Source: CAD feature listing. Evaluate the final solid. Frame: model axes, mm. Give positions to 0.01 mm unless a question says otherwise; leave off trailing zeros. Order: outer loops, then holes, each group sorted by start corner. A loop starts at its lowest first (then second) coordinate and runs counter-clockwise, first axis right, second up. Notation, with made-up numbers: M 89.5,39 L 139.5,39 A17 cw 139.5,61 Z; hole C 6.25,-26.5 d1. An arc over 180 degrees is marked long. Answer in a Markdown table with one row per item. Add a question column.
(1) Section query C-C, the plane x = 6.25. Return loops of the section in (y, z).
(2) Mould query, pull axis X, two halves, no side actions, for faces 1 (the face through (4, 1, 0)), 2 (the face through (4, 2.54, -2)), 3 (the face through (0, 1, -2)). Classes: pulls with the +X half, pulls with the -X half, needs draft (parallel to the pull), parting line crosses it, or undercut.
(3) Section query A-A, the plane y = 4.5. Return loops of the section in (x, z), plus the area to 3 significant figures.
(4) Pin query (flat end, axial travel): P1, Ø0.7, axis at y = 4, z = -1, coming from the -X side; P2, Ø0.7, axis at y = 6.5, z = -3.5, coming from the +X side; P3, Ø1.5, axis at x = 6, y = 3, coming from the +Z side; P4, Ø3, axis at x = 3, y = 6.5, coming from the +Z side. Return the tip coordinate at first contact, or that it passes through.
(5) Material intervals for line 1 along X through (y, z) = (6.5, -3.4); line 2 along Y through (x, z) = (6.75, -3.1), sorted ascending.
(6) Section query D-D, the plane x = 4.25. Return loops of the section in (y, z), plus the area to 3 significant figures.
(7) Section query B-B, the plane z = -1.15. Return loops of the section in (x, y), plus the area to 3 significant figures.
from build123d import *
from OCP.BRepFilletAPI import BRepFilletAPI_MakeChamfer

# Parameters (mm, degrees)
SKETCH1_W                   = 7.62
SKETCH1_H                   = 4.826
BOSS_EXTRUDE1_DEPTH         = 2.54
SKETCH2_W                   = 0.635
SKETCH2_H                   = 0.635
BOSS_EXTRUDE2_DEPTH         = 5.842
CHAMFER2_SIZE               = 0.1524
CHAMFER2_SIZE2              = 0.071065287
CHAMFER1_SIZE               = 0.254
LPATTERN2_COUNT             = 3
LPATTERN2_PITCH             = 2.54
LPATTERN2_COUNT_DIR2        = 2
LPATTERN2_PITCH_DIR2        = 2.54
CHAMFER2_OF_LPATTERN2_SIZE  = 0.1524
CHAMFER2_OF_LPATTERN2_SIZE2 = 0.071065287


with BuildPart() as part:
    # Sketch1 → Boss-Extrude1 (new body)
    with BuildSketch(Plane(origin=(0, 0, 0), x_dir=(1, 0, 0), z_dir=(0, 1, 0))):
        with Locations((3.81, 2.413)):
            Rectangle(SKETCH1_W, SKETCH1_H)
    extrude(amount=BOSS_EXTRUDE1_DEPTH)

    # Sketch2 → Boss-Extrude2 (add)
    with BuildSketch(Plane(origin=(0, 2.54, 0), x_dir=(1, 0, 0), z_dir=(0, 1, 0))):
        with Locations((1.27, 1.143)):
            Rectangle(SKETCH2_W, SKETCH2_H)
    boss_extrude2 = extrude(amount=BOSS_EXTRUDE2_DEPTH)

    # Chamfer2: one chamfer whose edges measure the first distance from different faces: ONE call of the kernel's chamfer builder (chamfer() names one face for all edges)
    chamfer2_edges_1 = [part.edges().sort_by_distance(p)[0] for p in [
        (1.5875, 8.382, -1.143),
    ]]
    chamfer2_side_1 = [part.faces().sort_by_distance(p)[0] for p in [
        (1.5875, 5.461, -1.143),
    ]]
    chamfer2_edges_2 = [part.edges().sort_by_distance(p)[0] for p in [
        (1.27, 8.382, -1.4605),
    ]]
    chamfer2_side_2 = [part.faces().sort_by_distance(p)[0] for p in [
        (1.27, 5.461, -1.4605),
    ]]
    chamfer2_edges_3 = [part.edges().sort_by_distance(p)[0] for p in [
        (0.9525, 8.382, -1.143),
    ]]
    chamfer2_side_3 = [part.faces().sort_by_distance(p)[0] for p in [
        (0.9525, 5.461, -1.143),
    ]]
    chamfer2_edges_4 = [part.edges().sort_by_distance(p)[0] for p in [
        (1.27, 8.382, -0.8255),
    ]]
    chamfer2_side_4 = [part.faces().sort_by_distance(p)[0] for p in [
        (1.27, 5.461, -0.8255),
    ]]
    chamfer2 = BRepFilletAPI_MakeChamfer(part.part.solid().wrapped)
    for e in chamfer2_edges_1:
        chamfer2.Add(CHAMFER2_SIZE, CHAMFER2_SIZE2, e.wrapped, chamfer2_side_1[0].wrapped)  # the first distance lies on this face
    for e in chamfer2_edges_2:
        chamfer2.Add(CHAMFER2_SIZE, CHAMFER2_SIZE2, e.wrapped, chamfer2_side_2[0].wrapped)  # the first distance lies on this face
    for e in chamfer2_edges_3:
        chamfer2.Add(CHAMFER2_SIZE, CHAMFER2_SIZE2, e.wrapped, chamfer2_side_3[0].wrapped)  # the first distance lies on this face
    for e in chamfer2_edges_4:
        chamfer2.Add(CHAMFER2_SIZE, CHAMFER2_SIZE2, e.wrapped, chamfer2_side_4[0].wrapped)  # the first distance lies on this face
    add(Compound.cast(chamfer2.Shape()), mode=Mode.REPLACE)

    # Chamfer1
    chamfer1_edges = [part.edges().sort_by_distance(p)[0] for p in [
        (0, 1.27, -4.826),
        (7.62, 1.27, -4.826),
        (7.62, 1.27, 0),
        (0, 1.27, 0),
    ]]
    chamfer(chamfer1_edges, length=CHAMFER1_SIZE)

    # LPattern2: Boss-Extrude2 3 × 2
    with Locations(*[(i * LPATTERN2_PITCH, 0, -j * LPATTERN2_PITCH_DIR2) for i in range(LPATTERN2_COUNT) for j in range(LPATTERN2_COUNT_DIR2) if (i, j) != (0, 0)]):
        add(boss_extrude2)

    # Chamfer2 of LPattern2: one chamfer whose edges measure the first distance from different faces: ONE call of the kernel's chamfer builder (chamfer() names one face for all edges)
    chamfer2_of_lpattern2_edges_1 = [part.edges().sort_by_distance(p)[0] for p in [
        (1.5875, 8.382, -3.683),
    ]]
    chamfer2_of_lpattern2_side_1 = [part.faces().sort_by_distance(p)[0] for p in [
        (1.5875, 5.461, -3.683),
    ]]
    chamfer2_of_lpattern2_edges_2 = [part.edges().sort_by_distance(p)[0] for p in [
        (1.27, 8.382, -4.0005),
    ]]
    chamfer2_of_lpattern2_side_2 = [part.faces().sort_by_distance(p)[0] for p in [
        (1.27, 5.461, -4.0005),
    ]]
    chamfer2_of_lpattern2_edges_3 = [part.edges().sort_by_distance(p)[0] for p in [
        (0.9525, 8.382, -3.683),
    ]]
    chamfer2_of_lpattern2_side_3 = [part.faces().sort_by_distance(p)[0] for p in [
        (0.9525, 5.461, -3.683),
    ]]
    chamfer2_of_lpattern2_edges_4 = [part.edges().sort_by_distance(p)[0] for p in [
        (1.27, 8.382, -3.3655),
    ]]
    chamfer2_of_lpattern2_side_4 = [part.faces().sort_by_distance(p)[0] for p in [
        (1.27, 5.461, -3.3655),
    ]]
    chamfer2_of_lpattern2_edges_5 = [part.edges().sort_by_distance(p)[0] for p in [
        (4.1275, 8.382, -1.143),
    ]]
    chamfer2_of_lpattern2_side_5 = [part.faces().sort_by_distance(p)[0] for p in [
        (4.1275, 5.461, -1.143),
    ]]
    chamfer2_of_lpattern2_edges_6 = [part.edges().sort_by_distance(p)[0] for p in [
        (3.81, 8.382, -1.4605),
    ]]
    chamfer2_of_lpattern2_side_6 = [part.faces().sort_by_distance(p)[0] for p in [
        (3.81, 5.461, -1.4605),
    ]]
    chamfer2_of_lpattern2_edges_7 = [part.edges().sort_by_distance(p)[0] for p in [
        (3.4925, 8.382, -1.143),
    ]]
    chamfer2_of_lpattern2_side_7 = [part.faces().sort_by_distance(p)[0] for p in [
        (3.4925, 5.461, -1.143),
    ]]
    chamfer2_of_lpattern2_edges_8 = [part.edges().sort_by_distance(p)[0] for p in [
        (3.81, 8.382, -0.8255),
    ]]
    chamfer2_of_lpattern2_side_8 = [part.faces().sort_by_distance(p)[0] for p in [
        (3.81, 5.461, -0.8255),
    ]]
    chamfer2_of_lpattern2_edges_9 = [part.edges().sort_by_distance(p)[0] for p in [
        (4.1275, 8.382, -3.683),
    ]]
    chamfer2_of_lpattern2_side_9 = [part.faces().sort_by_distance(p)[0] for p in [
        (4.1275, 5.461, -3.683),
    ]]
    chamfer2_of_lpattern2_edges_10 = [part.edges().sort_by_distance(p)[0] for p in [
        (3.81, 8.382, -4.0005),
    ]]
    chamfer2_of_lpattern2_side_10 = [part.faces().sort_by_distance(p)[0] for p in [
        (3.81, 5.461, -4.0005),
    ]]
    chamfer2_of_lpattern2_edges_11 = [part.edges().sort_by_distance(p)[0] for p in [
        (3.4925, 8.382, -3.683),
    ]]
    chamfer2_of_lpattern2_side_11 = [part.faces().sort_by_distance(p)[0] for p in [
        (3.4925, 5.461, -3.683),
    ]]
    chamfer2_of_lpattern2_edges_12 = [part.edges().sort_by_distance(p)[0] for p in [
        (3.81, 8.382, -3.3655),
    ]]
    chamfer2_of_lpattern2_side_12 = [part.faces().sort_by_distance(p)[0] for p in [
        (3.81, 5.461, -3.3655),
    ]]
    chamfer2_of_lpattern2_edges_13 = [part.edges().sort_by_distance(p)[0] for p in [
        (6.6675, 8.382, -1.143),
    ]]
    chamfer2_of_lpattern2_side_13 = [part.faces().sort_by_distance(p)[0] for p in [
        (6.6675, 5.461, -1.143),
    ]]
    chamfer2_of_lpattern2_edges_14 = [part.edges().sort_by_distance(p)[0] for p in [
        (6.35, 8.382, -1.4605),
    ]]
    chamfer2_of_lpattern2_side_14 = [part.faces().sort_by_distance(p)[0] for p in [
        (6.35, 5.461, -1.4605),
    ]]
    chamfer2_of_lpattern2_edges_15 = [part.edges().sort_by_distance(p)[0] for p in [
        (6.0325, 8.382, -1.143),
    ]]
    chamfer2_of_lpattern2_side_15 = [part.faces().sort_by_distance(p)[0] for p in [
        (6.0325, 5.461, -1.143),
    ]]
    chamfer2_of_lpattern2_edges_16 = [part.edges().sort_by_distance(p)[0] for p in [
        (6.35, 8.382, -0.8255),
    ]]
    chamfer2_of_lpattern2_side_16 = [part.faces().sort_by_distance(p)[0] for p in [
        (6.35, 5.461, -0.8255),
    ]]
    chamfer2_of_lpattern2_edges_17 = [part.edges().sort_by_distance(p)[0] for p in [
        (6.6675, 8.382, -3.683),
    ]]
    chamfer2_of_lpattern2_side_17 = [part.faces().sort_by_distance(p)[0] for p in [
        (6.6675, 5.461, -3.683),
    ]]
    chamfer2_of_lpattern2_edges_18 = [part.edges().sort_by_distance(p)[0] for p in [
        (6.35, 8.382, -4.0005),
    ]]
    chamfer2_of_lpattern2_side_18 = [part.faces().sort_by_distance(p)[0] for p in [
        (6.35, 5.461, -4.0005),
    ]]
    chamfer2_of_lpattern2_edges_19 = [part.edges().sort_by_distance(p)[0] for p in [
        (6.0325, 8.382, -3.683),
    ]]
    chamfer2_of_lpattern2_side_19 = [part.faces().sort_by_distance(p)[0] for p in [
        (6.0325, 5.461, -3.683),
    ]]
    chamfer2_of_lpattern2_edges_20 = [part.edges().sort_by_distance(p)[0] for p in [
        (6.35, 8.382, -3.3655),
    ]]
    chamfer2_of_lpattern2_side_20 = [part.faces().sort_by_distance(p)[0] for p in [
        (6.35, 5.461, -3.3655),
    ]]
    chamfer2_of_lpattern2 = BRepFilletAPI_MakeChamfer(part.part.solid().wrapped)
    for e in chamfer2_of_lpattern2_edges_1:
        chamfer2_of_lpattern2.Add(CHAMFER2_OF_LPATTERN2_SIZE, CHAMFER2_OF_LPATTERN2_SIZE2, e.wrapped, chamfer2_of_lpattern2_side_1[0].wrapped)  # the first distance lies on this face
    for e in chamfer2_of_lpattern2_edges_2:
        chamfer2_of_lpattern2.Add(CHAMFER2_OF_LPATTERN2_SIZE, CHAMFER2_OF_LPATTERN2_SIZE2, e.wrapped, chamfer2_of_lpattern2_side_2[0].wrapped)  # the first distance lies on this face
    for e in chamfer2_of_lpattern2_edges_3:
        chamfer2_of_lpattern2.Add(CHAMFER2_OF_LPATTERN2_SIZE, CHAMFER2_OF_LPATTERN2_SIZE2, e.wrapped, chamfer2_of_lpattern2_side_3[0].wrapped)  # the first distance lies on this face
    for e in chamfer2_of_lpattern2_edges_4:
        chamfer2_of_lpattern2.Add(CHAMFER2_OF_LPATTERN2_SIZE, CHAMFER2_OF_LPATTERN2_SIZE2, e.wrapped, chamfer2_of_lpattern2_side_4[0].wrapped)  # the first distance lies on this face
    for e in chamfer2_of_lpattern2_edges_5:
        chamfer2_of_lpattern2.Add(CHAMFER2_OF_LPATTERN2_SIZE, CHAMFER2_OF_LPATTERN2_SIZE2, e.wrapped, chamfer2_of_lpattern2_side_5[0].wrapped)  # the first distance lies on this face
    for e in chamfer2_of_lpattern2_edges_6:
        chamfer2_of_lpattern2.Add(CHAMFER2_OF_LPATTERN2_SIZE, CHAMFER2_OF_LPATTERN2_SIZE2, e.wrapped, chamfer2_of_lpattern2_side_6[0].wrapped)  # the first distance lies on this face
    for e in chamfer2_of_lpattern2_edges_7:
        chamfer2_of_lpattern2.Add(CHAMFER2_OF_LPATTERN2_SIZE, CHAMFER2_OF_LPATTERN2_SIZE2, e.wrapped, chamfer2_of_lpattern2_side_7[0].wrapped)  # the first distance lies on this face
    for e in chamfer2_of_lpattern2_edges_8:
        chamfer2_of_lpattern2.Add(CHAMFER2_OF_LPATTERN2_SIZE, CHAMFER2_OF_LPATTERN2_SIZE2, e.wrapped, chamfer2_of_lpattern2_side_8[0].wrapped)  # the first distance lies on this face
    for e in chamfer2_of_lpattern2_edges_9:
        chamfer2_of_lpattern2.Add(CHAMFER2_OF_LPATTERN2_SIZE, CHAMFER2_OF_LPATTERN2_SIZE2, e.wrapped, chamfer2_of_lpattern2_side_9[0].wrapped)  # the first distance lies on this face
    for e in chamfer2_of_lpattern2_edges_10:
        chamfer2_of_lpattern2.Add(CHAMFER2_OF_LPATTERN2_SIZE, CHAMFER2_OF_LPATTERN2_SIZE2, e.wrapped, chamfer2_of_lpattern2_side_10[0].wrapped)  # the first distance lies on this face
    for e in chamfer2_of_lpattern2_edges_11:
        chamfer2_of_lpattern2.Add(CHAMFER2_OF_LPATTERN2_SIZE, CHAMFER2_OF_LPATTERN2_SIZE2, e.wrapped, chamfer2_of_lpattern2_side_11[0].wrapped)  # the first distance lies on this face
    for e in chamfer2_of_lpattern2_edges_12:
        chamfer2_of_lpattern2.Add(CHAMFER2_OF_LPATTERN2_SIZE, CHAMFER2_OF_LPATTERN2_SIZE2, e.wrapped, chamfer2_of_lpattern2_side_12[0].wrapped)  # the first distance lies on this face
    for e in chamfer2_of_lpattern2_edges_13:
        chamfer2_of_lpattern2.Add(CHAMFER2_OF_LPATTERN2_SIZE, CHAMFER2_OF_LPATTERN2_SIZE2, e.wrapped, chamfer2_of_lpattern2_side_13[0].wrapped)  # the first distance lies on this face
    for e in chamfer2_of_lpattern2_edges_14:
        chamfer2_of_lpattern2.Add(CHAMFER2_OF_LPATTERN2_SIZE, CHAMFER2_OF_LPATTERN2_SIZE2, e.wrapped, chamfer2_of_lpattern2_side_14[0].wrapped)  # the first distance lies on this face
    for e in chamfer2_of_lpattern2_edges_15:
        chamfer2_of_lpattern2.Add(CHAMFER2_OF_LPATTERN2_SIZE, CHAMFER2_OF_LPATTERN2_SIZE2, e.wrapped, chamfer2_of_lpattern2_side_15[0].wrapped)  # the first distance lies on this face
    for e in chamfer2_of_lpattern2_edges_16:
        chamfer2_of_lpattern2.Add(CHAMFER2_OF_LPATTERN2_SIZE, CHAMFER2_OF_LPATTERN2_SIZE2, e.wrapped, chamfer2_of_lpattern2_side_16[0].wrapped)  # the first distance lies on this face
    for e in chamfer2_of_lpattern2_edges_17:
        chamfer2_of_lpattern2.Add(CHAMFER2_OF_LPATTERN2_SIZE, CHAMFER2_OF_LPATTERN2_SIZE2, e.wrapped, chamfer2_of_lpattern2_side_17[0].wrapped)  # the first distance lies on this face
    for e in chamfer2_of_lpattern2_edges_18:
        chamfer2_of_lpattern2.Add(CHAMFER2_OF_LPATTERN2_SIZE, CHAMFER2_OF_LPATTERN2_SIZE2, e.wrapped, chamfer2_of_lpattern2_side_18[0].wrapped)  # the first distance lies on this face
    for e in chamfer2_of_lpattern2_edges_19:
        chamfer2_of_lpattern2.Add(CHAMFER2_OF_LPATTERN2_SIZE, CHAMFER2_OF_LPATTERN2_SIZE2, e.wrapped, chamfer2_of_lpattern2_side_19[0].wrapped)  # the first distance lies on this face
    for e in chamfer2_of_lpattern2_edges_20:
        chamfer2_of_lpattern2.Add(CHAMFER2_OF_LPATTERN2_SIZE, CHAMFER2_OF_LPATTERN2_SIZE2, e.wrapped, chamfer2_of_lpattern2_side_20[0].wrapped)  # the first distance lies on this face
    add(Compound.cast(chamfer2_of_lpattern2.Shape()), mode=Mode.REPLACE)


solid = part.part
Values follow:
| question | item | result |
|---|---|---|
| 1 | outline | M 0,-4.83 L 2.54,-4.83 L 2.54,-4 L 8.23,-4 L 8.38,-3.93 L 8.38,-3.44 L 8.23,-3.37 L 2.54,-3.37 L 2.54,-1.46 L 8.23,-1.46 L 8.38,-1.39 L 8.38,-0.9 L 8.23,-0.83 L 2.54,-0.83 L 2.54,0 L 0,0 Z |
| 2 | face 1 | needs draft |
| 2 | face 2 | undercut |
| 2 | face 3 | pulls with the -X half |
| 3 | outline | M 0.95,-4 L 1.59,-4 L 1.59,-3.37 L 0.95,-3.37 Z; M 0.95,-1.46 L 1.59,-1.46 L 1.59,-0.83 L 0.95,-0.83 Z; M 3.49,-4 L 4.13,-4 L 4.13,-3.37 L 3.49,-3.37 Z; M 3.49,-1.46 L 4.13,-1.46 L 4.13,-0.83 L 3.49,-0.83 Z; M 6.03,-4 L 6.67,-4 L 6.67,-3.37 L 6.03,-3.37 Z; M 6.03,-1.46 L 6.67,-1.46 L 6.67,-0.83 L 6.03,-0.83 Z |
| 3 | area | 2.42 mm² |
| 4 | P1 | stops at x = 0.95 |
| 4 | P2 | stops at x = 6.67 |
| 4 | P3 | stops at z = 0 |
| 4 | P4 | stops at z = -0.83 |
| 5 | line 1 | x = 0.95 to 1.59, 3.49 to 4.13, 6.03 to 6.67 |
| 5 | line 2 | y = 0 to 2.54 |
| 6 | outline | M 0,-4.83 L 2.54,-4.83 L 2.54,0 L 0,0 Z |
| 6 | area | 12.3 mm² |
| 7 | outline | M 0,0 L 7.62,0 L 7.62,2.54 L 6.67,2.54 L 6.67,8.23 L 6.6,8.38 L 6.1,8.38 L 6.03,8.23 L 6.03,2.54 L 4.13,2.54 L 4.13,8.23 L 4.06,8.38 L 3.56,8.38 L 3.49,8.23 L 3.49,2.54 L 1.59,2.54 L 1.59,8.23 L 1.52,8.38 L 1.02,8.38 L 0.95,8.23 L 0.95,2.54 L 0,2.54 Z |
| 7 | area | 30.5 mm² |
